Read the model definition and answer for the solid it produces. Units are mm, in the model's axes. A direction names the side the tool comes from. Coordinates: 2 decimals unless noted, no trailing zeros. Write each loop counter-clockwise with the first axis right and the second up, starting at its lowest first coordinate (ties: lowest second). Pieces come first, ordered by that corner, then holes. Notation, with made-up numbers: M -28.5,9 L 24.5,9 A32 ccw 24.5,45 Z; hole C 81,87 d6. An arc over 180 degrees is marked long. Write item = value, one per line.
from build123d import *

# Parameters (mm, degrees)
POCKET_DEPTH       = 70.9409245757
POCKET_DEPTH_BACK  = 63.6409245757
POLARPATTERN_COUNT = 5


with BuildPart() as part:
    # Sketch → Revolution (revolve)
    with BuildSketch(Plane.XY):
        Polygon((3.25, 5.4), (1.3, 5.4), (1.3, -1.9), (10.95, -1.9), (10.95, -0.4), (3.25, -0.4), align=None)
    revolve(axis=Axis((0, 0, 0), (0, 1, 0)))

    # Sketch002 (on Face3 of Revolution) → Pocket (cut, two sides)
    with BuildSketch(Plane.XZ.offset(1.9)) as pocket_sk:
        with BuildLine():
            Line((1.4964773799, 10.847260274), (2.8231817433, 5.526139709))
            ThreePointArc((2.8231817433, 5.526139709), (3.3969474543, 4.6754970609), (4.3832600433, 4.392676477))
            Line((4.3832600433, 4.392676477), (9.8539206254, 4.7752223308))
            ThreePointArc((9.8539206254, 4.7752223308), (6.4362485126, 8.8587360884), (1.4964773799, 10.847260274))
        make_face()
    pocket = extrude(amount=-POCKET_DEPTH, mode=Mode.SUBTRACT) + extrude(pocket_sk.sketch, amount=POCKET_DEPTH_BACK, mode=Mode.SUBTRACT)

    # PolarPattern: Pocket ×5 about axis
    polarpattern_axis = Axis((0, -1.9, 0), (0, -1, 0))
    for i in range(1, POLARPATTERN_COUNT):
        add(pocket.rotate(polarpattern_axis, i * 360 / POLARPATTERN_COUNT), mode=Mode.SUBTRACT)


solid = part.part
Item 1: Find section D-D (x = 2.25). Determine the outline of the cut face in (y, z), and give its area (3 significant figures).
Worked answers:
outline = M -1.9,-7.21 L -0.4,-7.21 L -0.4,-2.35 L 5.4,-2.35 L 5.4,2.35 L -0.4,2.35 L -0.4,7.83 L -1.9,7.83 Z
area = 49.8 mm²
Item 2: Consider line 1 along Z through (x, y) = (0, 0); line 2 along Y through (x, z) = (4.5, 1). Determine where each line is inside the solid, lowest interval first. Write a range as from..to.
Worked answers:
line_1 = -3.25..-1.3, 1.3..3.25
line_2 = -1.9..-0.4
Item 3: For a pull along Z with two mould halves and no side action, classify faces 1 (the face through (5.5, -1.16, -1.77)), 2 (the face through (3.094, -1.16, -7.917)), 3 (the face through (-0.02, -1.14, 10.95)) as released by +Z, released by -Z, zero draft, split by the parting line, or undercut.
Worked answers:
face_1 = undercut
face_2 = released by -Z
face_3 = released by +Z
Item 4: Find section A-A (x = 0). Determine the outline of the cut face in (y, z), and give its area (3 significant figures).
Worked answers:
outline = M -1.9,-5.78 L -0.4,-5.78 L -0.4,-3.25 L 5.4,-3.25 L 5.4,-1.3 L -1.9,-1.3 Z; M -1.9,1.3 L 5.4,1.3 L 5.4,3.25 L -0.4,3.25 L -0.4,10.95 L -1.9,10.95 Z
area = 43.8 mm²
Item 5: Which of the six approach directions +Z, -Z, +X, -X, +Y, -Y give full straight-line access (tool end or side, diameter ignored) to faces 4 (the face through (-3.04, -1.16, -7.87)), 5 (the face through (-6.42, -1.14, -8.87)), 6 (the face through (-6.574, -1.16, -5.389)), 7 (the face through (8.49, -1.16, 0.5)), 8 (the face through (7.08, -1.16, 4.58))?
Worked answers:
face_4 = -Z, +Y, -Y
face_5 = -Z, -X, +Y, -Y
face_6 = -X, +Y, -Y
face_7 = +X, +Y, -Y
face_8 = +Z, +Y, -Y
Item 6: Find section C-C (y = 1). Determine the outline of the cut face in (x, z), and give its area (3 significant figures).
Worked answers:
outline = C 0,0 d6.5; hole C 0,0 d2.6
area = 27.9 mm²
Item 7: A flat-ended cylindrical pin translates along its axis: pin 1 (2.5 mm diameter, centred on x = 0, z = 0, fed in from +Y). Find the tip coordinate at first contact, or state that the pin passes through.
Worked answers:
pin_1 = through
Item 8: Find section B-B (z = 0). Determine the outline of the cut face in (x, y).
Worked answers:
outline = M -7.69,-1.9 L -1.3,-1.9 L -1.3,5.4 L -3.25,5.4 L -3.25,-0.4 L -7.69,-0.4 Z; M 1.3,-1.9 L 7.69,-1.9 L 7.69,-0.4 L 3.25,-0.4 L 3.25,5.4 L 1.3,5.4 Z
